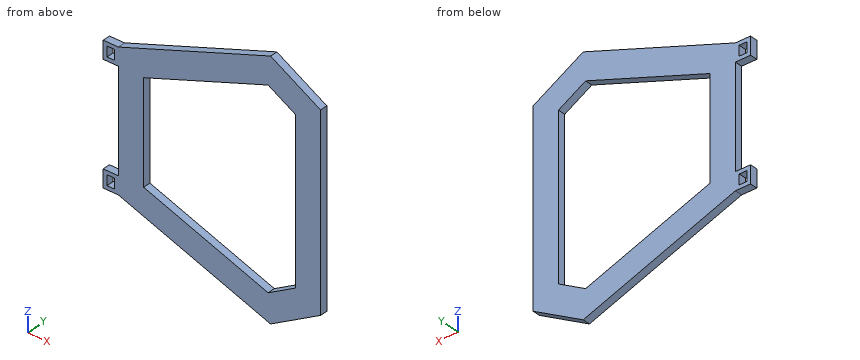
```python
from build123d import *

# Parameters (mm, degrees)
BOSS_EXTRUDE1_DEPTH = 3
BOSS_EXTRUDE2_DEPTH = 83
CUT_EXTRUDE1_DEPTH  = 81
SKETCH8_W           = 6
SKETCH8_H           = 7
SKETCH8_W_2         = 3
SKETCH8_H_2         = 4
BOSS_EXTRUDE4_DEPTH = 3


with BuildPart() as part:
    # Sketch2 → Boss-Extrude1 (new body)
    with BuildSketch(Plane(origin=(0, 0, 0), x_dir=(0, 0, -1), z_dir=(0, -1, 0))):
        Polygon((-37.5, 0), (37.5, 0), (48.918945144, -19.778193158), (27, -80), (-27, -80), (-48.918945144, -19.778193158), align=None)
        Polygon((-31.726497308, -10), (31.726497308, -10), (37.927152815, -20.739850379), (19.997924618, -70), (-19.997924618, -70), (-37.927152815, -20.739850379), align=None, mode=Mode.SUBTRACT)
    extrude(amount=BOSS_EXTRUDE1_DEPTH)

    # Sketch8 → Boss-Extrude4 (add)
    # profile 1 of 2: a face of its own
    with BuildSketch(Plane(origin=(0, 0, 0), x_dir=(1, 0, 0), z_dir=(0, 1, 0))):
        with Locations((-83, 23.5)):
            Rectangle(SKETCH8_W, SKETCH8_H)
        with Locations((-83, 23.5)):
            Rectangle(SKETCH8_W_2, SKETCH8_H_2, mode=Mode.SUBTRACT)
    # profile 2 of 2: a face of its own
    with BuildSketch(Plane(origin=(0, 0, 0), x_dir=(1, 0, 0), z_dir=(0, 1, 0))):
        with Locations((-83, -23.5)):
            Rectangle(SKETCH8_W, SKETCH8_H)
        with Locations((-83, -23.5)):
            Rectangle(SKETCH8_W_2, SKETCH8_H_2, mode=Mode.SUBTRACT)
    extrude(amount=-BOSS_EXTRUDE4_DEPTH)


with BuildPart() as body_2:
    # Sketch3 → Boss-Extrude2 (new body)
    with BuildSketch(Plane(origin=(-95, 0, 0), x_dir=(0, -1, 0), z_dir=(-1, 0, 0))):
        Polygon((13, 27), (0, 27), (0, -27), (13, -27), (13, -24), (3, -24), (3, 24), (13, 24), align=None)
    extrude(amount=BOSS_EXTRUDE2_DEPTH)

    # Sketch4 → Cut-Extrude1 (cut)
    with BuildSketch(Plane(origin=(-178, 0, 0), x_dir=(0, -1, 0), z_dir=(-1, 0, 0))):
        Polygon((2, 27), (1, 27), (1, 25), (2, 25), (4.25, 25), (4.25, 26), (2, 26), align=None)
        Polygon((4.25, -26), (2, -26), (2, -27), (1, -27), (1, -25), (2, -25), (4.25, -25), align=None)
    extrude(amount=-CUT_EXTRUDE1_DEPTH, mode=Mode.SUBTRACT)


solid = part.part
```
Design review of the part built by this model. Coordinates are the model's own, in mm. Give positions to 0.01 mm unless a question says otherwise; leave off trailing zeros. Write each loop counter-clockwise with the first axis right and the second up, starting at its lowest first coordinate (ties: lowest second). Pieces come first, ordered by that corner, then holes. Notation, with made-up numbers: (74, 11.5) - (133, 11.5) arc R17 ccw to (133, 37.5) - close; hole circle Ø5 at (30, 34.5). An arc over 180 degrees is marked (long way). Return JSON: item names as keys, results as strings. Group by question number.
(1) We need section B-B, the plane z = 17. Give the boundary of the cut face in (x, y), then the cut area to 3 significant figures.
(2) We need section A-A, the plane y = -1. Give the boundary of the cut face in (x, z), then the cut area to 3 significant figures.
(3) We need section C-C, the plane x = -35. Give the boundary of the cut face in (y, z).
(4) To check wall thickness, follow probe 1 along X at (y, z) = (-2.7, 3); probe 2 along Z at (x, y) = (-65.5, -2.3); probe 3 along Z at (x, y) = (-22.5, -0.4). State the ranges of each line that lie inside material, in increasing order.
(5) Insertion check: pin 1 (0.9 mm diameter, centred on y = -1, z = 23, fed in from +X); pin 2 (1.5 mm diameter, centred on x = -83.5, y = -2, fed in from -Z); pin 3 (1.5 mm diameter, centred on x = -83.5, y = -1, fed in from +Z). Each pin has a flat end and moves straight along its axis. Give the tip position at first contact, or say it passes through.
Reported:
{
 "1": {"outline": "(-80, -3) - (-70, -3) - (-70, 0) - (-80, 0) - close; (-10, -3) - (0, -3) - (0, 0) - (-10, 0) - close", "area": "60.0 mm2"},
 "2": {"outline": "(-86, -27) - (-80, -27) - (-19.78, -48.92) - (0, -37.5) - (0, 37.5) - (-19.78, 48.92) - (-80, 27) - (-86, 27) - (-86, 20) - (-80, 20) - (-80, -20) - (-86, -20) - close; hole (-84.5, -25.5) - (-81.5, -25.5) - (-81.5, -21.5) - (-84.5, -21.5) - close; hole (-84.5, 21.5) - (-81.5, 21.5) - (-81.5, 25.5) - (-84.5, 25.5) - close; hole (-70, -20) - (-20.74, -37.93) - (-10, -31.73) - (-10, 31.73) - (-20.74, 37.93) - (-70, 20) - close", "area": "2,740 mm2"},
 "3": {"outline": "(-3, -43.38) - (0, -43.38) - (0, -32.74) - (-3, -32.74) - close; (-3, 32.74) - (0, 32.74) - (0, 43.38) - (-3, 43.38) - close"},
 "4": {"probe 1": "x = -80 to -70, -10 to 0", "probe 2": "z = -32.28 to -21.64, 21.64 to 32.28", "probe 3": "z = -47.93 to -37.29, 37.29 to 47.93"},
 "5": {"pin 1": "stops at x = 0", "pin 2": "stops at z = -27", "pin 3": "stops at z = 27"}
}
